Source: CAD feature listing. Evaluate the final solid. Frame: model axes, mm. Face numbers are marked on the shaded views. A direction names the side the tool comes from. Round coordinates to 2 decimals unless told otherwise and drop trailing zeros. Order: outer loops, then holes, each group sorted by start corner. A loop starts at its lowest first (then second) coordinate and runs counter-clockwise, first axis right, second up. Notation, with made-up numbers: (-10.75, 14) -> (40.25, 14) arc R21 ccw to (40.25, 49) -> close; hole circle Ø3 at (62.25, 3). An arc over 180 degrees is marked (long way). Write item = value, one per line. Start each with the question number.
(1) Cut plane C-C on y = 0. Return the cut outline in (x, z).
(2) Cut plane B-B on x = 0. Return the cut outline in (y, z), then the cut area to 3 significant figures.
(3) Reachability of the marked faces 4 and 5 from +Z, -Z, +X, -X, +Y, -Y: full face, straight path, thin tool, end or side. Return the list, or none.
(4) Ray query, line 1 (X direction, y = 1.5, z = 101.5); line 2 (Y direction, x = 0, z = 81); line 3 (Y direction, x = -41, z = 79). Return the intervals inside material, ascending.
(5) Cut plane A-A on z = 52. Return the cut outline in (x, y), then the cut area to 3 significant figures.
(6) Contact query for flat-ended pins moving along their axis: pin 1 Ø6 at (y, z) = (-15.5, 85) entering from +X; pin 2 Ø12 at (y, z) = (1, 53.5) entering from -X; pin 3 Ø1.5 at (y, z) = (4, 58.5) entering from +X. Output: stop coordinate, or through.
(7) Draft query along X for the marked faces 1, 2 and 3. Return one class per face: released by +X, released by -X, zero draft, split by the parting line, or undercut.
(8) Cut plane D-D on x = -115. Return the cut outline in (y, z), then the cut area to 3 significant figures.
from build123d import *

# Parameters (mm, degrees)
SKETCH1_W           = 102.973663886
SKETCH1_H           = 10.457969277
SKETCH1_R           = 15
SKETCH1_R_2         = 10
BOSS_EXTRUDE1_DEPTH = 108


with BuildPart() as part:
    # Sketch1 → Boss-Extrude1 (new body)
    # profile 1 of 3: a face of its own
    with BuildSketch(Plane.XY):
        with Locations((-87.513168057, -16.191787915)):
            Rectangle(SKETCH1_W, SKETCH1_H)
    # profile 2 of 3: a face of its own
    with BuildSketch(Plane.XY):
        with BuildLine():
            Line((-36.026336114, -10.962803276), (-36.026336114, -21.420772553))
            ThreePointArc((-36.026336114, -21.420772553), (-13.958524045, -20.528091864), (6.914894743, -13.311056709))
            ThreePointArc((6.914894743, -13.311056709), (-9.740834476, -11.406846352), (-14.229640926, 4.745241735))
            ThreePointArc((-14.229640926, 4.745241735), (-22.592809035, -6.626630029), (-36.026336114, -10.962803276))
        make_face()
    # profile 3 of 3: a face of its own
    with BuildSketch(Plane.XY):
        Circle(SKETCH1_R)
        Circle(SKETCH1_R_2, mode=Mode.SUBTRACT)
    extrude(amount=BOSS_EXTRUDE1_DEPTH)


solid = part.part
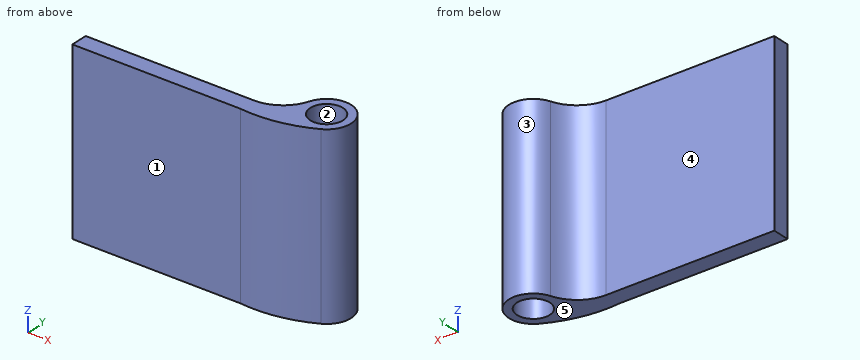
Evaluation:
q1.outline = (-16.44, 0) -> (-10, 0) -> (-10, 108) -> (-16.44, 108) -> close; (10, 0) -> (15, 0) -> (15, 108) -> (10, 108) -> close
q2.outline = (-16.47, 0) -> (-10, 0) -> (-10, 108) -> (-16.47, 108) -> close; (10, 0) -> (15, 0) -> (15, 108) -> (10, 108) -> close
q2.area = 1,240 mm^2
q3.face_4 = +Z, -Z, -X, +Y
q3.face_5 = -Z, +X, -X, +Y, -Y
q4.line_1 = -15.6 to -9.89, 9.89 to 14.92
q4.line_2 = -16.47 to -10, 10 to 15
q4.line_3 = -21.42 to -10.96
q5.outline = (-139, -21.42) -> (-36.03, -21.42) arc R75.79 ccw to (6.91, -13.31) arc R15 ccw (long way) to (-14.23, 4.75) arc R22.98 cw to (-36.03, -10.96) -> (-139, -10.96) -> close; hole circle Ø20 at (0, 0)
q5.area = 1,880 mm^2
q6.pin_1 = 8.29
q6.pin_2 = -20.58
q6.pin_3 = 14.64
q7.face_1 = zero draft
q7.face_2 = undercut
q7.face_3 = split by the parting line
q8.outline = (-21.42, 0) -> (-10.96, 0) -> (-10.96, 108) -> (-21.42, 108) -> close
q8.area = 1,130 mm^2
